Study the drawing (mm; zero at the part's minimum x, y, z) and answer. A direction names the side the tool comes from. Round coordinates to 2 decimals unless told otherwise and drop trailing zeros. Loops run counter-clockwise (first coordinate to the right, second up) from the corner with the lowest first, then second, coordinate; pieces in that order, holes last. Notation, with made-up numbers: (9, 15.5) - (19, 15.5) arc R26 cw to (19, 44.5) - close; hole circle Ø2 at (-21, 74.5). An arc over 180 degrees is marked (long way). Use CSV: the item, a comma, the result in double quotes. Start each with the question number.
1. Find section A-A (z = 124). Give the vertices of the cut face in (x, y), and give its area (3 significant figures).
2. Given pin 1 Ø3 at (y, z) = (1430, 587.5) entering from -X; pin 2 Ø5 at (y, z) = (1404.5, 533) entering from +X, each flat-ended and moving along its own axis, determine where each tip first touches the part or whether it passes through.
3. Find section D-D (y = 1905). Give the vertices of the cut face in (x, z).
4. Find section C-C (x = 819). Give the vertices of the cut face in (y, z), and give its area (3 significant figures).
5. Determine the mould class of the marked faces 4, 5, 6 and 7 for opening direction Y: +Y half, -Y half, draft (parallel to the pull), parting line (faces both ways), or undercut.
6. Consider line 1 along Y through (x, z) = (571.5, 957.5); line 2 along Z through (x, y) = (114, 1905); line 3 along Z through (x, y) = (722.5, 196). Determine where each line is inside the solid, lowest interval first.
7. Find section B-B (y = 381). Give the vertices of the cut face in (x, z).
8. A tool of negligible diameter and unlimited length cuts with its end or side. For the marked faces 1, 2 and 3, from which of +Z, -Z, +X, -X, +Y, -Y can it reach the whole face along a straight path? Write none if from no direction.
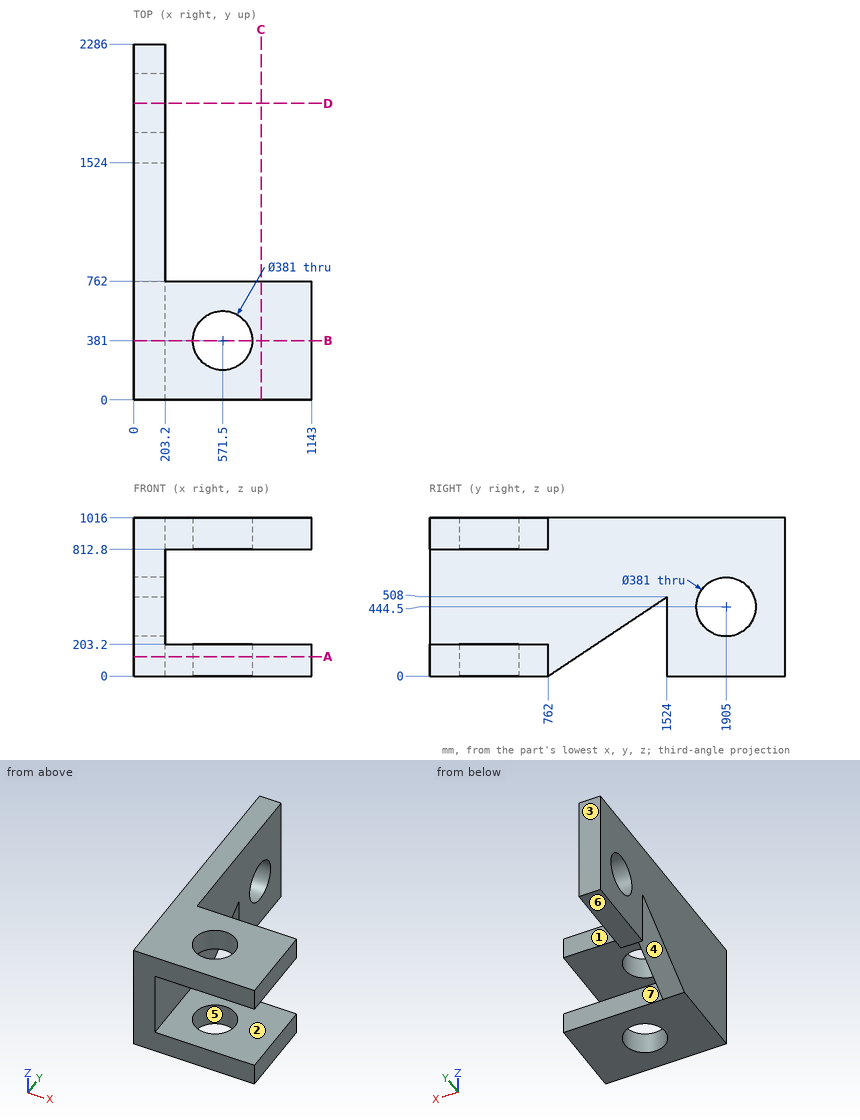
Filled sheet:
1,outline,"(0, 0) - (1143, 0) - (1143, 762) - (203.2, 762) - (203.2, 948) - (0, 948) - close; (0, 1524) - (203.2, 1524) - (203.2, 2286) - (0, 2286) - close; hole circle Ø381 at (571.5, 381)"
1,area,"950,000 mm²"
2,pin 1,"stops at x = 0"
2,pin 2,"stops at x = 203.2"
3,outline,"(0, 0) - (203.2, 0) - (203.2, 254) - (0, 254) - close; (0, 635) - (203.2, 635) - (203.2, 1016) - (0, 1016) - close"
4,outline,"(0, 0) - (762, 0) - (762, 203.2) - (0, 203.2) - close; (0, 812.8) - (762, 812.8) - (762, 1016) - (0, 1016) - close"
4,area,"310,000 mm²"
5,face 4,"undercut"
5,face 5,"undercut"
5,face 6,"draft"
5,face 7,"+Y half"
6,line 1,"y = 0 to 190.5, 571.5 to 762"
6,line 2,"z = 0 to 254, 635 to 1016"
6,line 3,"z = 0 to 203.2, 812.8 to 1016"
7,outline,"(0, 0) - (381, 0) - (381, 203.2) - (203.2, 203.2) - (203.2, 812.8) - (381, 812.8) - (381, 1016) - (0, 1016) - close; (762, 0) - (1143, 0) - (1143, 203.2) - (762, 203.2) - close; (762, 812.8) - (1143, 812.8) - (1143, 1016) - (762, 1016) - close"
8,face 1,"+Z, -Z, +X, +Y"
8,face 2,"+X, +Y, -Y"
8,face 3,"+Z, -Z, +X, -X, +Y"
